Study the drawing (mm; zero at the part's minimum x, y, z) and answer. A direction names the side the tool comes from. Give positions to 0.01 mm unless a question says otherwise; leave off trailing zeros. Loops run counter-clockwise (first coordinate to the right, second up) from the corner with the lowest first, then second, coordinate; pieces in that order, holes last. Notation, with made-up numbers: M 51,47 L 60,47 A23 cw 60,78 Z; hole C 61,2.25 d4. An arc over 180 degrees is marked long. Return JSON: item names as keys, results as strings.
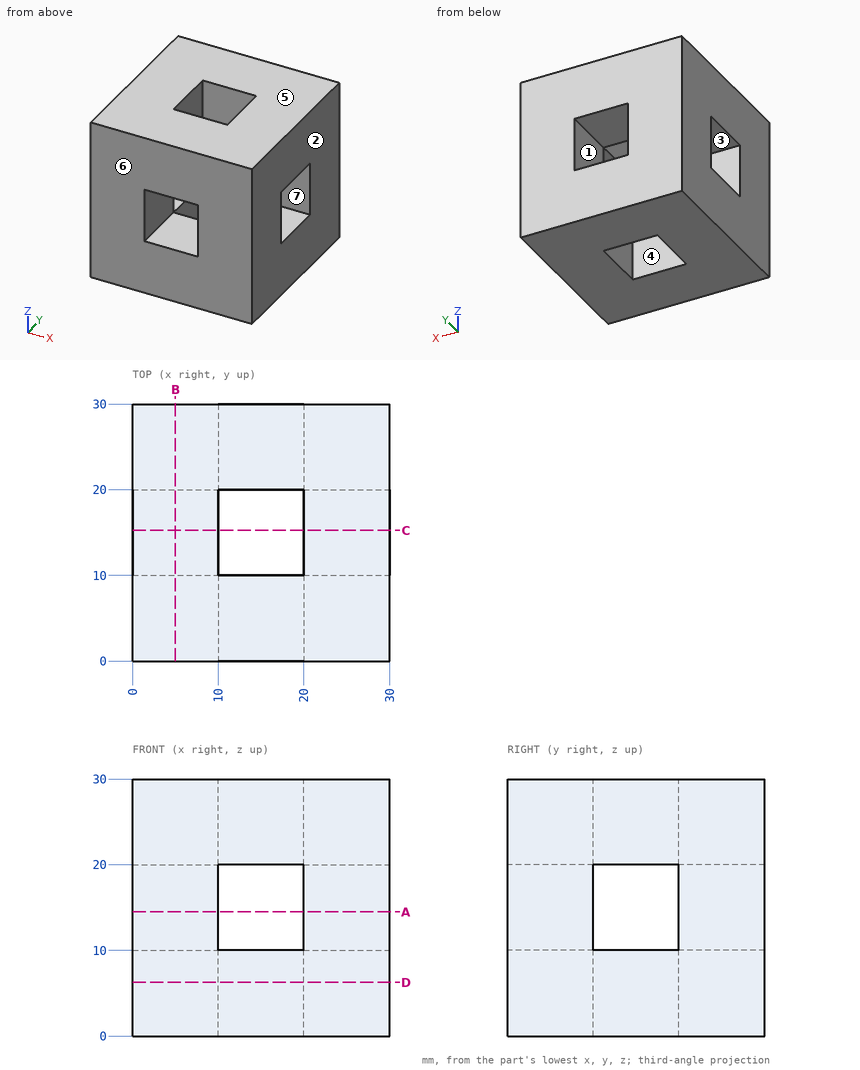
(1) The part is cut by section A-A (z = 14.5). Determine the outline of the cut face in (x, y).
Values follow:
{"outline": "M 0,0 L 10,0 L 10,10 L 0,10 Z; M 0,20 L 10,20 L 10,30 L 0,30 Z; M 20,0 L 30,0 L 30,10 L 20,10 Z; M 20,20 L 30,20 L 30,30 L 20,30 Z"}
(2) The part is cut by section B-B (x = 5). Determine the outline of the cut face in (y, z), and give its area (3 significant figures).
Values follow:
{"outline": "M 0,0 L 30,0 L 30,30 L 0,30 Z; hole M 10,10 L 20,10 L 20,20 L 10,20 Z", "area": "800 mm²"}
(3) A straight line is drawn through the part: line 1 along Y through (x, z) = (4.5, 11). Find the intervals that lie inside material, in ascending order.
Values follow:
{"line 1": "0 to 10, 20 to 30"}
(4) A tool of negligible diameter and unlimited length cuts with its end or side. For the marked faces 1, 2, 3 and 4, from which of +Z, -Z, +X, -X, +Y, -Y can it reach the whole face along a straight path? Write none if from no direction.
Values follow:
{"face 1": "+Y, -Y", "face 2": "+Z, -Z, +X, +Y, -Y", "face 3": "+X, -X", "face 4": "+Z, -Z"}
(5) Determine the mould class of the marked faces 5, 6 and 7 for opening direction Z: released by +Z, released by -Z, zero draft, split by the parting line, or undercut.
Values follow:
{"face 5": "released by +Z", "face 6": "zero draft", "face 7": "undercut"}
